Here's how the part is built. I have some questions about the finished solid (model axes, mm). Face numbers are marked on the shaded views. A direction names the side the tool comes from. Coordinates: 2 decimals unless noted, no trailing zeros. Loops run counter-clockwise (first coordinate to the right, second up) from the corner with the lowest first, then second, coordinate; pieces in that order, holes last. Notation, with made-up numbers: M -13,73 L 5,73 A19 ccw 5,107 Z; hole C 20,10.5 d9. An arc over 180 degrees is marked long. Use one line per item in the form item = value. Start each with the question number.
(1) Will this pin go through, and if not, where does the flat tip stop? P1, Ø6, axis at x = -7, z = 20.5, coming from the -Y side.
(2) Please list where these lines run through material, in increasing order: L1, parallel to Z at x = 0, y = -0.5; L2, parallel to Y at x = 4.5, z = 27; L3, parallel to X at y = 12.25, z = 4.
(3) Imagine slicing it at C-C, the plane y = -7.75. Please give me the cut outline in (x, z).
(4) Thinking about a two-plate mould opening in Z: for the marked faces 1, 2 and 3, which applies, +Z half, -Z half, draft (parallel to the pull), parting line (faces both ways), or undercut?
(5) Imagine slicing it at D-D, the plane y = -4.75. State how many separate pieces and enclosed holes the cut face has, and give its area (3 significant figures).
(6) On a 3-axis mill with a long thin cutter (end or side, diameter ignored), from which of +Z, -Z, +X, -X, +Y, -Y can I reach the whole of each face in a straight line? I mean the marked faces 4 and 5. Say none if no direction works.
(7) Imagine slicing it at B-B, the plane z = 7. Please give me the cut outline in (x, y).
(8) Imagine slicing it at A-A, the plane x = 0. Please give me the cut outline in (y, z), and give its area (3 significant figures).
```python
from build123d import *

# Parameters (mm, degrees)
F0_W     = 24
F0_H     = 26.5
F1_DEPTH = 29
F3_DEPTH = 25
F4_R     = 4.15
F5_DEPTH = 31
F6_R     = 1
F7_R     = 0.5


with BuildPart() as f1:
    # F0 (on Top) → F1 (new body)
    with BuildSketch(Plane.XY):
        Rectangle(F0_W, F0_H)
    extrude(amount=F1_DEPTH)

    # F2 (on face) → F3 (cut)
    with BuildSketch(Plane.YZ.offset(12)):
        Polygon((-6.75, 20), (-6.75, 29), (-13.25, 29), (-13.25, 16), (-2.75, 16), align=None)
    extrude(amount=-F3_DEPTH, mode=Mode.SUBTRACT)

    # F4 (on face) → F5 (cut)
    with BuildSketch(Plane.XZ.offset(13.25)):
        with Locations((0, 7)):
            Circle(F4_R)
    extrude(amount=-F5_DEPTH, mode=Mode.SUBTRACT)

    # F6
    f6_edges = [f1.edges().sort_by_distance(p)[0] for p in [
        (12, 0, 0),
        (12, 13.25, 14.5),
        (12, 3.25, 29),
        (12, -6.75, 24.5),
        (12, -4.75, 18),
        (12, -8, 16),
        (12, -13.25, 8),
        (-12, 0, 0),
        (-12, -13.25, 8),
        (-12, -8, 16),
        (-12, -4.75, 18),
        (-12, -6.75, 24.5),
        (-12, 3.25, 29),
        (-12, 13.25, 14.5),
        (0, -6.75, 29),
        (0, 13.25, 29),
        (0, 13.25, 0),
        (0, -13.25, 0),
        (0, -13.25, 16),
    ]]
    fillet(f6_edges, radius=F6_R)

    # F7
    f7_edges = [f1.edges().sort_by_distance(p)[0] for p in [
        (-4.15, 13.25, 7),
        (-4.15, -13.25, 7),
    ]]
    fillet(f7_edges, radius=F7_R)


solid = f1.part
```
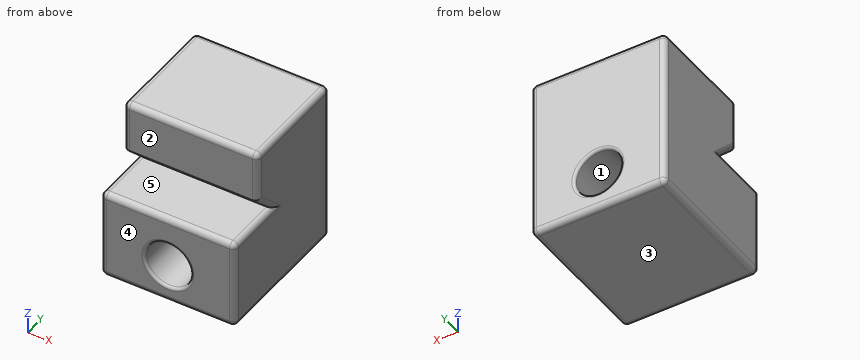
Answer:
q1.P1 = -6.75
q2.L1 = 0 to 2.85, 11.15 to 29
q2.L2 = -6.75 to 13.25
q2.L3 = -12 to -2.87, 2.87 to 12
q3.outline = M -12,1 A1 ccw -11,0 L 11,0 A1 ccw 12,1 L 12,15 A1 ccw 11,16 L -11,16 A1 ccw -12,15 Z; hole C 0,7 d8.3
q4.face_1 = undercut
q4.face_2 = draft
q4.face_3 = -Z half
q5.separate_pieces = 2
q5.enclosed_holes = 1
q5.area = 592 mm²
q6.face_4 = +Z, -Z, +X, -X, -Y
q6.face_5 = +X, -X, -Y
q7.outline = M -12,-12.25 A1 ccw -11,-13.25 L -4.65,-13.25 A0.5 ccw -4.15,-12.75 L -4.15,12.75 A0.5 ccw -4.65,13.25 L -11,13.25 A1 ccw -12,12.25 Z; M 4.15,-12.75 A0.5 ccw 4.65,-13.25 L 11,-13.25 A1 ccw 12,-12.25 L 12,12.25 A1 ccw 11,13.25 L 4.65,13.25 A0.5 ccw 4.15,12.75 Z
q8.outline = M -13.25,1 A1 ccw -12.25,0 L 12.25,0 A1 ccw 13.25,1 L 13.25,2.35 A0.5 ccw 12.75,2.85 L -12.75,2.85 A0.5 ccw -13.25,2.35 Z; M -13.25,11.65 A0.5 ccw -12.75,11.15 L 12.75,11.15 A0.5 ccw 13.25,11.65 L 13.25,28 A1 ccw 12.25,29 L -5.75,29 A1 ccw -6.75,28 L -6.75,20 L -2.75,16 L -12.25,16 A1 ccw -13.25,15 Z
q8.area = 455 mm²
